Part model, mm, in its own coordinate system. A direction names the side the tool comes from. Round coordinates to 2 decimals unless told otherwise and drop trailing zeros. Loops run counter-clockwise (first coordinate to the right, second up) from the corner with the lowest first, then second, coordinate; pieces in that order, holes last.
(1) Cut at D-D on z = -43.5. List the corners of the cut face in (x, y) (3 decimals), then the cut area to 3 significant figures.
(2) Tool access for faces 5 (the face through (0, 2, -46.5)), 6 (the face through (-4, 2, 0)), 7 (the face through (19.375, 2, -24)), 8 (the face through (1.65, 2, -20)), 9 (the face through (-13.83, 1.5, 2.52)): list every direction of +Z, -Z, +X, -X, +Y, -Y with a clear straight run to the whole face (end or side of a thin tool).
(3) Cut at A-A on z = -7.5. List the corners of the cut face in (x, y) (3 decimals).
(4) Flat gauge pins, fed straight in: pin 1 (2 mm diameter, centred on x = -12, z = -43.5, fed in from -Y); pin 2 (1.5 mm diameter, centred on x = 15.5, y = 1, fed in from +Z); pin 3 (1.5 mm diameter, centred on x = 3.5, y = 1, fed in from +Z); pin 4 (0.9 mm diameter, centred on x = -15, y = 1, fed in from +Z). Where does each tip first touch, or does it go through?
(5) Probe probe 1 along X at (y, z) = (1.25, -43.5) (3 decimals); probe 2 along X at (y, z) = (0.55, -36) (3 decimals); probe 3 along Z at (x, y) = (-12, 1.85). List the from-to ranges inside material, lowest first.
(6) Mould opens along Z. For faces 1 (the face through (-16, 2, 0)), 2 (the face through (5, 3.05, -21)), 3 (the face through (5, 2, 0)), 4 (the face through (-10, 2, 5)) say: +Z half, -Z half, draft (parallel to the pull), parting line (faces both ways), or undercut.
(7) Cut at B-B on x = 12. List the corners of the cut face in (y, z), then the cut area to 3 significant figures.
(8) Cut at C-C on y = 1.6. List the corners of the cut face in (x, z) (3 decimals), then the cut area to 3 significant figures.
from build123d import *

# Parameters (mm, degrees)
BOSS_EXTRUDE1_DEPTH      = 3.05
FILLET1_R                = 0.5
SKETCH3_W                = 3.3
SKETCH3_H                = 40
SKETCH3_H_2              = 1
CUT_EXTRUDE2_DEPTH       = 51.467248043
M3_TAPPED_DAMPER_HOLES_D = 2.5


with BuildPart() as part:
    # Sketch1 → Boss-Extrude1 (new body)
    with BuildSketch(Plane(origin=(0, 0, 0), x_dir=(1, 0, 0), z_dir=(0, 1, 0))):
        Polygon((-19.375, 0), (-19.375, 46.5), (19.375, 46.5), (19.375, 0), (12.375, 0), (15.261751346, -5), (5.261751346, -5), (8.148502692, 0), (-8.148502692, 0), (-5.261751346, -5), (-15.261751346, -5), (-12.375, 0), align=None)
    extrude(amount=BOSS_EXTRUDE1_DEPTH)

    # Fillet1
    fillet1_edges = [part.edges().sort_by_distance(p)[0] for p in [
        (12.375, 1.525, 0),
        (15.261751346, 1.525, 5),
        (5.261751346, 1.525, 5),
        (8.148502692, 1.525, 0),
        (-8.148502692, 1.525, 0),
        (-5.261751346, 1.525, 5),
        (-15.261751346, 1.525, 5),
        (-12.375, 1.525, 0),
    ]]
    fillet(fillet1_edges, radius=FILLET1_R)

    # Sketch3 → Cut-Extrude2 (cut, through all)
    with BuildSketch(Plane(origin=(0, 3.05, 0), x_dir=(1, 0, 0), z_dir=(0, 1, 0))):
        with Locations((0, 20)):
            Rectangle(SKETCH3_W, SKETCH3_H)
        with Locations((0, -1.7)):
            Rectangle(SKETCH3_W, SKETCH3_H_2)
    extrude(amount=-CUT_EXTRUDE2_DEPTH, mode=Mode.SUBTRACT)

    # M3 Tapped Damper Holes (through all)
    with Locations(Plane(origin=(0, 3.05, 0), x_dir=(1, 0, 0), z_dir=(0, 1, 0))):
        with Locations((-12, 43.5), (12, 43.5)):
            Hole(M3_TAPPED_DAMPER_HOLES_D / 2)


solid = part.part
Final values:
1. outline: (-19.375, 0) - (-13.25, 0) - (-13.25, 3.05) - (-19.375, 3.05) - close; (-10.75, 0) - (10.75, 0) - (10.75, 3.05) - (-10.75, 3.05) - close; (13.25, 0) - (19.375, 0) - (19.375, 3.05) - (13.25, 3.05) - close
1. area: 103 mm2
2. face 5: -Z, +X, -X, +Y, -Y
2. face 6: +Y, -Y
2. face 7: +Z, -Z, +X, +Y, -Y
2. face 8: +Z, +Y, -Y
2. face 9: -X, +Y, -Y
3. outline: (-19.375, 0) - (-1.65, 0) - (-1.65, 3.05) - (-19.375, 3.05) - close; (1.65, 0) - (19.375, 0) - (19.375, 3.05) - (1.65, 3.05) - close
4. pin 1: passes through
4. pin 2: stops at z = 4.85
4. pin 3: stops at z = 0
4. pin 4: stops at z = 4.98
5. probe 1: x = -19.375 to -13.25, -10.75 to 10.75, 13.25 to 19.375
5. probe 2: x = -19.375 to -1.65, 1.65 to 19.375
5. probe 3: z = -46.5 to -44.75, -42.25 to 5
6. face 1: undercut
6. face 2: draft
6. face 3: undercut
6. face 4: +Z half
7. outline: (0, -46.5) - (3.05, -46.5) - (3.05, -44.75) - (0, -44.75) - close; (0, -42.25) - (3.05, -42.25) - (3.05, 5) - (0, 5) - close
7. area: 149 mm2
8. outline: (-19.375, -46.5) - (19.375, -46.5) - (19.375, 0) - (13.241, 0) arc R0.5 cw to (12.808, 0.75) - (14.829, 4.25) arc R0.5 ccw to (14.396, 5) - (6.128, 5) arc R0.5 ccw to (5.695, 4.25) - (7.715, 0.75) arc R0.5 cw to (7.282, 0) - (1.65, 0) - (1.65, -40) - (-1.65, -40) - (-1.65, 0) - (-7.282, 0) arc R0.5 cw to (-7.715, 0.75) - (-5.695, 4.25) arc R0.5 ccw to (-6.128, 5) - (-14.396, 5) arc R0.5 ccw to (-14.829, 4.25) - (-12.808, 0.75) arc R0.5 cw to (-13.241, 0) - (-19.375, 0) - close; hole circle Ø2.5 at (-12, -43.5); hole circle Ø2.5 at (12, -43.5)
8. area: 1,730 mm2
